Check sheet for the modelled part. Datum: model origin and axes. Units: mm. Give positions to 0.01 mm unless a question says otherwise; leave off trailing zeros. Loops run counter-clockwise (first coordinate to the right, second up) from the corner with the lowest first, then second, coordinate; pieces in that order, holes last.
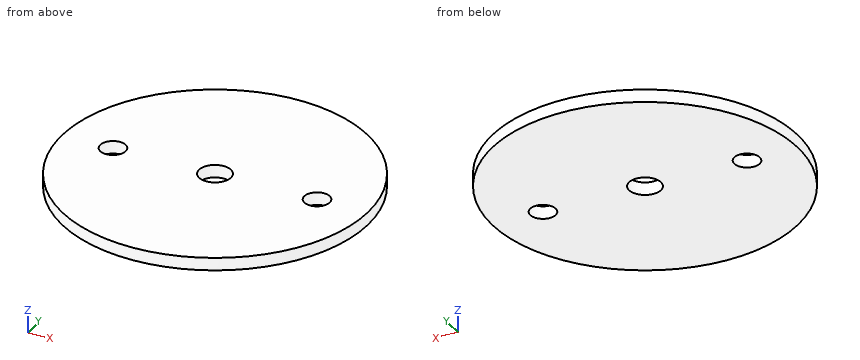
```python
from build123d import *

# Parameters (mm, degrees)
SKETCH1_R                          = 38.1
BOSS_EXTRUDE1_DEPTH                = 1.5875
F_1_4_0_25_DIAMETER_HOLE1_D        = 6.35
F_5_16_0_3125_DIAMETER_HOLE1_D     = 7.9375
F_5_16_0_3125_DIAMETER_HOLE1_DEPTH = 3.302


with BuildPart() as part:
    # Sketch1 → Boss-Extrude1 (new body, symmetric)
    with BuildSketch(Plane.XY):
        Circle(SKETCH1_R)
    extrude(amount=BOSS_EXTRUDE1_DEPTH, both=True)

    # 1/4 (0.25) Diameter Hole1 (through all)
    with Locations(Plane.XY.offset(1.5875)):
        with Locations((-25.4, 0), (25.4, 0)):
            Hole(F_1_4_0_25_DIAMETER_HOLE1_D / 2)

    # 5/16 (0.3125) Diameter Hole1
    with Locations(Plane.XY.offset(1.5875)):
        with Locations((0, 0)):
            Hole(F_5_16_0_3125_DIAMETER_HOLE1_D / 2, depth=F_5_16_0_3125_DIAMETER_HOLE1_DEPTH)


solid = part.part
```
(1) Gauge pin test, flat ends, axial feed: pin 1 Ø7 at (x, y) = (0, 0) entering from -Z; pin 2 Ø1 at (y, z) = (8, 0) entering from -X; pin 3 Ø10 at (x, y) = (25.4, 0) entering from -Z; pin 4 Ø1.5 at (y, z) = (24.5, 0.5) entering from -X. Record the tip position at first contact, or that the pin passes through.
(2) Section check C-C on z = 0.45. Give the number of separate pieces and of enclosed holes in the cut face, plus the area to 3 significant figures.
(3) Section check B-B on y = 0. Record the boundary of the cut face in (x, z) (1 decimal), plus the area to 3 significant figures.
(4) Material ranges on line 1 (X direction, y = -2, z = -1.1); line 2 (X direction, y = 1.5, z = -1.1); line 3 (Y direction, x = -11.5, z = -0.45), recorded low to high.
(5) Section check A-A on x = 0. Record the boundary of the cut face in (y, z).
(6) Section check D-D on x = -25.4. Record the boundary of the cut face in (y, z) (1 decimal), plus the area to 3 significant figures.
Computed values:
1. pin 1: passes through
1. pin 2: stops at x = -37.35
1. pin 3: stops at z = -1.59
1. pin 4: stops at x = -29.79
2. separate pieces: 1
2. enclosed holes: 3
2. area: 4,450 mm2
3. outline: (-38.1, -1.6) - (-28.6, -1.6) - (-28.6, 1.6) - (-38.1, 1.6) - close; (-22.2, -1.6) - (-4, -1.6) - (-4, 1.6) - (-22.2, 1.6) - close; (4, -1.6) - (22.2, -1.6) - (22.2, 1.6) - (4, 1.6) - close; (28.6, -1.6) - (38.1, -1.6) - (38.1, 1.6) - (28.6, 1.6) - close
3. area: 176 mm2
4. line 1: x = -38.05 to -27.87, -22.93 to -3.43, 3.43 to 22.93, 27.87 to 38.05
4. line 2: x = -38.07 to -28.2, -22.6 to -3.67, 3.67 to 22.6, 28.2 to 38.07
4. line 3: y = -36.32 to 36.32
5. outline: (-38.1, -1.59) - (-3.97, -1.59) - (-3.97, 1.59) - (-38.1, 1.59) - close; (3.97, -1.59) - (38.1, -1.59) - (38.1, 1.59) - (3.97, 1.59) - close
6. outline: (-28.4, -1.6) - (-3.2, -1.6) - (-3.2, 1.6) - (-28.4, 1.6) - close; (3.2, -1.6) - (28.4, -1.6) - (28.4, 1.6) - (3.2, 1.6) - close
6. area: 160 mm2
